CAD build for the part. Positions are in the model's coordinates, mm. A direction names the side the tool comes from. Coordinates: 2 decimals unless noted, no trailing zeros. Write each loop counter-clockwise with the first axis right and the second up, starting at its lowest first coordinate (ties: lowest second). Pieces come first, ordered by that corner, then holes.
```python
from build123d import *

# Parameters (mm, degrees)
SKETCH1_W           = 100
SKETCH1_H           = 100
BOSS_EXTRUDE1_DEPTH = 226
SKETCH5_W           = 150
SKETCH5_H           = 10
CUT_EXTRUDE2_DEPTH  = 125
SKETCH6_W           = 15
SKETCH6_H           = 15
CUT_EXTRUDE3_DEPTH  = 125
CUT_EXTRUDE6_DEPTH  = 7.5
BOSS_EXTRUDE2_DEPTH = 6.5


with BuildPart() as part:
    # Sketch1 → Boss-Extrude1 (new body)
    with BuildSketch(Plane(origin=(0, 0, 0), x_dir=(1, 0, 0), z_dir=(0, 1, 0))):
        Rectangle(SKETCH1_W, SKETCH1_H)
    extrude(amount=BOSS_EXTRUDE1_DEPTH)

    # Sketch5 → Cut-Extrude2 (cut)
    with BuildSketch(Plane(origin=(50, 0, -50), x_dir=(0, -1, 0), z_dir=(-0.707106781, 0, 0.707106781))):
        with Locations((-113, -5)):
            Rectangle(SKETCH5_W, SKETCH5_H)
        with Locations((-113, 5)):
            Rectangle(SKETCH5_W, SKETCH5_H)
    extrude(amount=CUT_EXTRUDE2_DEPTH, mode=Mode.SUBTRACT)

    # Sketch6 → Cut-Extrude3 (cut)
    with BuildSketch(Plane(origin=(-50, 0, 50), x_dir=(0.707106781, 0, 0.707106781), z_dir=(-0.707106781, 0, 0.707106781))):
        with Locations((0, 113)):
            Rectangle(SKETCH6_W, SKETCH6_H)
    extrude(amount=-CUT_EXTRUDE3_DEPTH, mode=Mode.SUBTRACT)

    # Sketch8 → Cut-Extrude6 (cut)
    with BuildSketch(Plane.XY.offset(50)):
        with BuildLine():
            Line((-39.393398282, 114), (-39.393398282, 112))
            Line((-39.393398282, 112), (-5, 112))
            Line((-5, 112), (-2.291287847, 112))
            ThreePointArc((-2.291287847, 112), (2.5, 113), (-2.291287847, 114))
            Line((-2.291287847, 114), (-5, 114))
            Line((-5, 114), (-39.393398282, 114))
        make_face()
    extrude(amount=-CUT_EXTRUDE6_DEPTH, mode=Mode.SUBTRACT)

    # Sketch10 → Boss-Extrude2 (add)
    with BuildSketch(Plane.XY.offset(50)):
        with BuildLine():
            ThreePointArc((-0.472805429, 113.162650012), (0.407016588, 113.290409189), (0, 112.5))
            Line((0, 112.5), (0, 111.5))
            ThreePointArc((0, 111.5), (1.221049764, 113.871227567), (-1.418416287, 113.487950036))
            ThreePointArc((-1.418416287, 113.487950036), (-1.780506402, 112.700361849), (-2.291287847, 112))
            ThreePointArc((-2.291287847, 112), (-1.928903385, 111.409612711), (-1.418416287, 110.941336541))
            ThreePointArc((-1.418416287, 110.941336541), (-0.906091719, 112.03517002), (-0.472805429, 113.162650012))
        make_face()
    extrude(amount=-BOSS_EXTRUDE2_DEPTH)


solid = part.part
```
Item 1: Which spindle directions (+Z, -Z, +X, -X, +Y, -Y) get a long thin tool onto all of the face, cutting with end or side? Do faces 5 (the flat face through (-36.283, 108.704, 46.89)), 6 (the flat face through (-17, 112, 46)), 7 (the flat face through (50, 111, 1)), 8 (the flat face through (-4.23, 114.05, -9.91)). Say none if no direction does.
Item 2: Wall check: line 1 along X through (y, z) = (113, 45); line 2 along Y through (x, z) = (-9, 16); line 3 along Z through (x, y) = (15.5, 187.5). Give the ranges that are in metal, low to high.
Item 3: Two-plate mould, pull along Z, no slides. Class faces 1 (the flat face through (-1, 111, -50)), 2 (the flat face through (-46.89, 112.895, 36.283)), 3 (the flat face through (6, 38, -7)), 4 (the flat face through (-1, 0, -1)): +Z half, -Z half, draft (parallel to the pull), parting line (faces both ways), or undercut.
Item 4: Saw through at A-A, the plane y = 58.5. Write the cut outline in (x, z), and give its area (3 significant figures).
Item 5: Saw through at B-B, the plane x = 6.5. Write the cut outline in (y, z).
Item 6: Saw through at C-C, the plane z = -4.5. Write the cut outline in (x, y), and give its area (3 significant figures).
Working result:
1. face 5: -X
1. face 6: +Z, -X
1. face 7: +Z, -Z, +X, +Y, -Y
1. face 8: none
2. line 1: x = -1.62 to -0.53, 0.5 to 1.5, 2.5 to 50
2. line 2: y = 0 to 38, 188 to 226
2. line 3: z = -50 to -29.64, -1.36 to 50
3. face 1: -Z half
3. face 2: +Z half
3. face 3: undercut
3. face 4: draft
4. outline: (-50, -50) - (35.86, -50) - (-45.46, 31.32) - (-31.32, 45.46) - (50, -35.86) - (50, 50) - (-50, 50) - close
4. area: 7,600 mm2
5. outline: (0, -50) - (226, -50) - (226, 50) - (0, 50) - close; hole (38, -20.64) - (188, -20.64) - (188, 7.64) - (38, 7.64) - close
6. outline: (-50, 0) - (50, 0) - (50, 226) - (-50, 226) - close; hole (-9.64, 38) - (18.64, 38) - (18.64, 188) - (-9.64, 188) - close
6. area: 18,400 mm2
